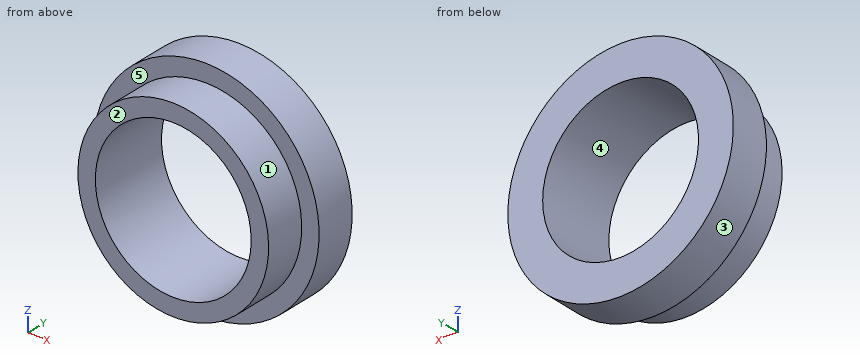
```python
from build123d import *

# Parameters (mm, degrees)
F0_W     = 12.7
F0_H     = 34.925
F0_H_2   = 29.5275
F3_R     = 24.13
F4_DEPTH = 25.4


with BuildPart() as f1:
    # F0 (on Right) → F1 (revolve)
    with BuildSketch(Plane.YZ):
        with Locations((6.35, -17.4625)):
            Rectangle(F0_W, F0_H)
    revolve(axis=Axis((0, 6.35, 0), (0, 1, 0)))

    # F0 (on Right) → F2 (revolve)
    with BuildSketch(Plane.YZ):
        with Locations((6.35, -17.4625)):
            Rectangle(F0_W, F0_H)
        with Locations((-6.35, 14.76375)):
            Rectangle(F0_W, F0_H_2)
    revolve(axis=Axis((0, 0, 0), (0, 1, 0)))

    # F3 (on face) → F4 (cut)
    with BuildSketch(Plane.XZ.offset(12.7)):
        Circle(F3_R)
    extrude(amount=-F4_DEPTH, mode=Mode.SUBTRACT)


solid = f1.part
```
Geometry check sheet. Reference: the model listing, model coordinates, mm. Face numbers are marked on the shaded views. A direction names the side the tool comes from. Coordinates: 2 decimals unless noted, no trailing zeros. Write each loop counter-clockwise with the first axis right and the second up, starting at its lowest first coordinate (ties: lowest second). Pieces come first, ordered by that corner, then holes. Notation, with made-up numbers: M 75,88.25 L 134,88.25 A12 ccw 134,100.25 Z; hole C 22.25,-21 d10. An arc over 180 degrees is marked long. One line per item, written item: value. Start each with the question number.
(1) Release check for a two-part mould opening along X. For the marked faces 3, 4 and 5 record: released by +X, released by -X, zero draft, split by the parting line, or undercut.
(2) Scan lines: line 1 along Z through (x, y) = (0, 1.75) (3 decimals); line 2 along Z through (x, y) = (-10.5, -9.75); line 3 along X through (y, z) = (3.25, 8.5). Record each from-to range of solid material in increasing order. Write a range as [from, to].
(3) Tool access check on the marked faces 1 and 2. Record the directions out of +Z, -Z, +X, -X, +Y, -Y that give a thin tool (end or side, any length) a straight path to the whole face; none if there is none.
(4) Sectioned sample at B-B, the plane x = 0. Enter the section's corners in (y, z) (1 decimal), and give its area (3 significant figures).
(5) Sectioned sample at A-A, the plane z = 0. Enter the section's corners in (x, y) (1 decimal).
(6) Sectioned sample at D-D, the plane x = 26. Enter the section's corners in (y, z).
(7) Depth check by flat-ended pin: pin 1 (1.5 mm diameter, centred on x = 13, y = 0.5, fed in from +Z); pin 2 (12 mm diameter, centred on y = 9.5, z = 11, fed in from +X); pin 3 (1 mm diameter, centred on x = 14.5, y = -5, fed in from -Z). Enter the tip coordinate at first touch or a pass-through.
(8) Sectioned sample at C-C, the plane y = -2.5. Enter the section's corners in (x, z) (1 decimal).
Filled sheet:
1. face 3: split by the parting line
1. face 4: undercut
1. face 5: zero draft
2. line 1: [-34.925, -24.13], [24.13, 34.925]
2. line 2: [-27.6, -21.73], [21.73, 27.6]
2. line 3: [-33.87, -22.58], [22.58, 33.87]
3. face 1: -Y
3. face 2: +Z, -Z, +X, -X, -Y
4. outline: M -12.7,-29.5 L 0,-29.5 L 0,-34.9 L 12.7,-34.9 L 12.7,-24.1 L -12.7,-24.1 Z; M -12.7,24.1 L 12.7,24.1 L 12.7,34.9 L 0,34.9 L 0,29.5 L -12.7,29.5 Z
4. area: 411 mm²
5. outline: M -34.9,0 L -29.5,0 L -29.5,-12.7 L -24.1,-12.7 L -24.1,12.7 L -34.9,12.7 Z; M 24.1,-12.7 L 29.5,-12.7 L 29.5,0 L 34.9,0 L 34.9,12.7 L 24.1,12.7 Z
6. outline: M -12.7,-14 L 0,-14 L 0,-23.32 L 12.7,-23.32 L 12.7,23.32 L 0,23.32 L 0,14 L -12.7,14 Z
7. pin 1: z = 32.71
7. pin 2: x = 34.57
7. pin 3: z = -26
8. outline: C 0,0 d59.1; hole C 0,0 d48.3
